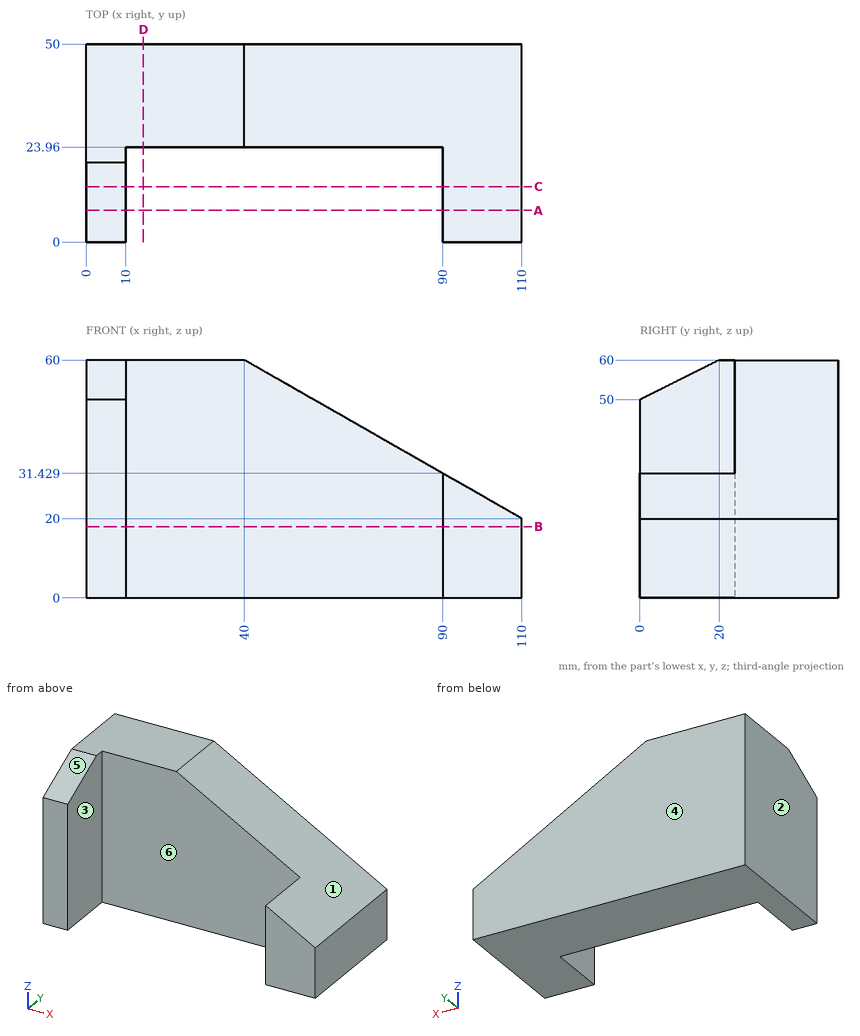
Geometry: see drawing. Coordinates: mm, zero at the bounding-box minimum. A direction names the side the tool comes from. Coordinates: 2 decimals unless noted, no trailing zeros. Write each loop counter-clockwise with the first axis right and the second up, starting at its lowest first coordinate (ties: lowest second). Pieces come first, ordered by that corner, then holes.
1) Section C-C on y = 14. Output: boundary loops of the cut face in (x, z).
2) Mould query, pull axis X, two halves, no side actions, for the marked faces 1, 2, 3 and 4. Classes: pulls with the +X half, pulls with the -X half, needs draft (parallel to the pull), parting line crosses it, or undercut.
3) Section B-B on z = 18. Output: boundary loops of the cut face in (x, y).
4) Set-up query: the marked faces 5 and 6. Return all of +Z, -Z, +X, -X, +Y, -Y with unobstructed straight access to the full face (end or side cutting, diameter ignored); none if empty.
5) Material intervals for line 1 along X through (y, z) = (4, 3); line 2 along Y through (x, z) = (17.5, 19); line 3 along X through (y, z) = (23.5, 33), sorted ascending.
6) Pin query (flat end, axial travel): pin 1 Ø2 at (x, z) = (23.5, 46.5) entering from -Y. Return the tip coordinate at first contact, or that it passes through.
7) Section A-A on y = 8. Output: boundary loops of the cut face in (x, z).
8) Section D-D on x = 14.5. Output: boundary loops of the cut face in (y, z).
Check result:
1. outline: (0, 0) - (10, 0) - (10, 57) - (0, 57) - close; (90, 0) - (110, 0) - (110, 20) - (90, 31.43) - close
2. face 1: pulls with the +X half
2. face 2: pulls with the -X half
2. face 3: undercut
2. face 4: needs draft
3. outline: (0, 0) - (10, 0) - (10, 23.96) - (90, 23.96) - (90, 0) - (110, 0) - (110, 50) - (0, 50) - close
4. face 5: +Z, +X, -X, -Y
4. face 6: +Z, -Z, -Y
5. line 1: x = 0 to 10, 90 to 110
5. line 2: y = 23.96 to 50
5. line 3: x = 0 to 10
6. pin 1: stops at y = 23.96
7. outline: (0, 0) - (10, 0) - (10, 54) - (0, 54) - close; (90, 0) - (110, 0) - (110, 20) - (90, 31.43) - close
8. outline: (23.96, 0) - (50, 0) - (50, 60) - (23.96, 60) - close
